For this review, take the finished solid that the model builds, in its own axes (mm). A direction names the side the tool comes from. Coordinates: 2 decimals unless noted, no trailing zeros. Write each loop counter-clockwise with the first axis right and the second up, starting at its lowest first coordinate (ties: lowest second). Pieces come first, ordered by that corner, then holes. Notation, with made-up numbers: M -2,16.5 L 30,16.5 A37 ccw 30,52.5 Z; hole C 23,79 d7. An arc over 180 degrees is marked long. One line per question, with ' | ' between items.
Autodesk Inventor part; units mm, degrees
ref_plane "Work Plane1" through (0, 0, -15) normal (0, 0, 1) x (1, 0, 0)
ref_plane "YZ Plane" through (0, 0, 0) normal (1, 0, 0) x (0, 1, 0)
ref_plane "XZ Plane" through (0, 0, 0) normal (0, 1, 0) x (-1, 0, 0)
sketch "Sketch1" plane through (0, 0, 0) normal (0, 0, 1) x (1, 0, 0)
  line L0 (0, 0) -> (25, 0)
  line L1 (25, 0) -> (25, 40)
  line L2 (25, 40) -> (0, 40)
  line L3 (0, 40) -> (0, 0)
  dimension "d1" = 25
  dimension "d2" = 40
  dimension "d3" = 25
extrude "Extrusion1" add sketch "Sketch1" against normal blind 30
sketch "Sketch2" plane through (25, 0, 0) normal (1, 0, 0) x (0, 0, -1)
  line L0 (0, 0) -> (30, 0)
  circle A0 centre (15, 6.56) radius 2.46
extrude "Extrusion2" cut sketch "Sketch2" against normal blind 30
sketch "Sketch3" plane through (0, 0, 0) normal (-1, 0, 0) x (0, 0, 1)
  line L0 (0, 0) -> (-30, 0)
  line L1 (-25.05, 0) -> (-4.95, 0)
  line L2 (-4.95, 0) -> (-4.95, 33.12)
  line L3 (-4.95, 33.12) -> (-25.05, 33.12)
  line L4 (-25.05, 33.12) -> (-25.05, 0)
  dimension "d11" = 20.1
extrude "Extrusion3" cut sketch "Sketch3" against normal blind 20
sketch "Sketch4" plane through (0, 0, 0) normal (0, -1, 0) x (1, 0, 0)
  line L0 (20, -4.95) -> (20, -25.05)
  line L1 (20, -15) -> (25, -15)
  line L2 (25, 0) -> (25, -30)
  line L3 (20, -8.025) -> (25, -8.025)
  line L4 (25, -8.025) -> (25, -21.975)
  line L5 (25, -21.975) -> (20, -21.975)
  line L6 (20, -21.975) -> (20, -8.025)
  line L7 (20, -8.025) -> (25, -21.975) construction
  line L8 (25, -8.025) -> (20, -21.975) construction
  line L9 (25, -12.54) -> (25, -17.46)
  point P0 (0, 0)
  point P1 (22.5, -15)
  dimension "d14" = 13.95
extrude "Extrusion4" add sketch "Sketch4" along normal blind 15
sketch "Sketch5" plane through (20, 0, 0) normal (-1, 0, 0) x (0, 0, 1)
  circle A0 centre (-15, 6.56) radius 2.46
  circle A1 centre (-15, 6.56) radius 4.7025
  circle A2 centre (-15, 6.56) radius 2.46
  circle A3 centre (-15, 6.56) radius 2.46
  point P0 (0, 0)
  dimension "d17" = 9.405
extrude "Extrusion5" cut sketch "Sketch5" against normal blind 2.1
sketch "Sketch6" plane through (25, 0, 0) normal (1, 0, 0) x (0, 0, -1)
  circle A0 centre (15, 6.56) radius 4.7025
  line L0 (15, 6.56) -> (15, 23.56)
  circle A1 centre (15, 23.56) radius 2.46
  point P0 (0, 0)
  dimension "d20" = 17
  dimension "d21" = 4.92
extrude "Extrusion6" cut sketch "Sketch6" against normal blind 10 contours A1
sketch "Sketch7" plane through (20, 0, 0) normal (-1, 0, 0) x (0, 0, 1)
  circle A0 centre (-15, 23.56) radius 2.46
  circle A1 centre (-15, 23.56) radius 4.7025
  point P0 (0, 0)
  dimension "d24" = 9.405
extrude "Extrusion7" cut sketch "Sketch7" against normal blind 2.1
sketch "Sketch9" plane through (25, 0, 0) normal (1, 0, 0) x (0, 0, -1)
  circle A0 centre (15, 6.56) radius 2.46
  circle A1 centre (15, 6.56) radius 2.46
  circle A2 centre (15, 23.56) radius 2.46
  circle A3 centre (15, 23.56) radius 2.46
  line L0 (30, 40) -> (30, 0)
  line L1 (30, 0) -> (30, 40)
  line L2 (30, 40) -> (0, 40)
  line L3 (0, 40) -> (0, 0)
  line L4 (0, 0) -> (8.025, 0)
  line L5 (21.975, 0) -> (21.975, -15)
  line L6 (21.975, -15) -> (8.025, -15)
  line L7 (8.025, -15) -> (8.025, 0)
  line L8 (0, 0) -> (8.025, 0)
  line L9 (21.975, 0) -> (30, 0)
extrude "Extrusion8" add sketch "Sketch9" along normal blind 5
sketch "Sketch10" plane through (0, 40, 0) normal (0, 1, 0) x (1, 0, 0)
  line L0 (0, 30) -> (30, 30)
  line L1 (30, 0) -> (0, 0)
  line L2 (0, 30) -> (30, 30)
  line L3 (30, 30) -> (30, 0)
  line L4 (30, 0) -> (0, 0)
  line L5 (0, 0) -> (0, 30)
extrude "Extrusion9" add sketch "Sketch10" along normal blind 30
sketch "Sketch12" plane through (30, 0, 0) normal (1, 0, 0) x (0, 0, -1)
  circle A0 centre (15, 6.56) radius 2.46
  line L0 (15, 6.56) -> (15, 15.06)
  circle A1 centre (15, 15.06) radius 2.525
  point P0 (0, 0)
  dimension "d31" = 8.5
  dimension "d33" = 5.05
extrude "Extrusion10" cut sketch "Sketch12" against normal blind 30 contours A1
sketch "Sketch14" plane through (0, 0, 0) normal (0, 0, 1) x (1, 0, 0)
  line L0 (30, 70) -> (0, 70)
  line L1 (0, 100) -> (-8, 100)
  line L2 (30, 0) -> (30, 70)
  line L3 (30, 118) -> (30, 70)
  line L4 (30, 105) -> (30, 100)
  line L5 (0, 70) -> (30, 70)
  line L6 (0, 70) -> (0, 100)
  line L7 (30, 122.5) -> (30, 118)
  line L8 (30, 70) -> (30, 145)
  line L9 (-2, 157.5) -> (-8, 160)
  line L10 (-2, 102.5) -> (-8, 100)
  line L11 (4, 130) -> (-2, 102.5)
  line L12 (4, 130) -> (-2, 157.5)
  line L13 (-8, 160) -> (15, 160)
  line L14 (30, 145) -> (15, 160)
  point P0 (0, 0)
  dimension "d47" = 30
extrude "Extrusion12" add sketch "Sketch14" against normal blind 30
sketch "Sketch15" plane through (0, 0, -25.05) normal (-1, 0, 0) x (0, 0, 1)
  line L0 (0, 33.12) -> (20.1, 33.12)
  line L1 (20.1, 33.12) -> (20.1, 0)
  line L2 (0, 33.12) -> (20.1, 33.12)
  line L3 (20.1, 33.12) -> (20.1, 31.1)
  line L4 (20.1, 31.1) -> (0, 31.1)
  line L5 (0, 31.1) -> (0, 33.12)
  point P0 (25.05, 0)
  dimension "d57" = 2.02
extrude "Extrusion13" add sketch "Sketch15" against normal blind 20
sketch "Sketch27" plane through (0, 0, 0) normal (0, 0, 1) x (1, 0, 0)
  point P0 (0, 0)
sketch "Sketch28" plane through (0, 0, 0) normal (0, 0, 1) x (1, 0, 0)
  line L0 (0, 100) -> (-8, 100)
  line L1 (0, 100) -> (-8, 100)
  line L2 (-8, 100) -> (-2, 102.5)
  line L3 (-8, 100) -> (-2, 102.5)
  line L4 (-2, 102.5) -> (4, 130)
  line L5 (-2, 102.5) -> (4, 130)
  line L6 (4, 130) -> (-2, 157.5)
  line L7 (4, 130) -> (-2, 157.5)
  line L8 (-2, 157.5) -> (-8, 160)
  line L9 (-2, 157.5) -> (-8, 160)
  line L10 (-8, 160) -> (15, 160)
  line L11 (-8, 160) -> (15, 160)
  line L12 (15, 160) -> (30, 145)
  line L13 (15, 160) -> (30, 145)
  line L14 (30, 145) -> (30, 93)
  line L15 (30, 0) -> (30, 145)
  line L16 (30, 93) -> (0, 93)
  line L17 (0, 0) -> (0, 100)
  line L18 (0, 93) -> (0, 100)
  dimension "d98" = 52
extrude "Extrusion14" add sketch "Sketch28" along normal blind 45
ref_plane "Work Plane1" through (0, 0, -15) normal (0, 0, 1) x (1, 0, 0)
mirror "Mirror1" about plane through (0, 0, -15) normal (0, 0, 1) of "Extrusion14"
properties part number "55mm_x_120mm"
1) We need section B-B on y = 6.56. State the section outline as (x, z) points.
Responses:
outline: M 0,-30 L 30,-30 L 30,-17.46 L 22.1,-17.46 L 22.1,-19.7 L 20,-19.7 L 20,-25.05 L 0,-25.05 Z; M 0,-4.95 L 20,-4.95 L 20,-10.3 L 22.1,-10.3 L 22.1,-12.54 L 30,-12.54 L 30,0 L 0,0 Z
2) To check wall thickness, follow line 1 along Z through (x, y) = (28.75, 23.56); line 2 along X through (y, z) = (75, -5.5); line 3 along Y through (x, z) = (14.5, -37). State the ranges of each line that lie inside material, in increasing order. Write a range as [from, to].
Responses:
line 1: [-30, -17.46], [-12.54, 0] | line 2: [0, 30] | line 3: [93, 160]
3) Machinability: for faces 4 (the flat face through (15, 47, -30)), 5 (the flat face through (15, 47, 0)), 6 (the flat face through (22.1, 21.5, -13)), 7 (the flat face through (-4.958, 101.268, -14.16)), 8 (the flat face through (20, 8, -20)), which of the approach directions +Z, -Z, +X, -X, +Y, -Y give a long, thin tool a straight path to every point of the face, cutting with its end or side? Answer none if there is none.
Responses:
face 4: -Z, +X, -X, -Y | face 5: +Z, +X, -X, -Y | face 6: -X | face 7: +Z, -Z, -X | face 8: -X, -Y
4) Insertion check: pin 1 Ø22 at (x, y) = (7.5, 17.5) entering from -Z; pin 2 Ø9 at (x, z) = (20.5, -2) entering from -Y; pin 3 Ø2 at (y, z) = (96, -61.5) entering from -X. Each pin has a flat end and moves straight along its axis. Give the tip position at first contact, or say it passes through.
Responses:
pin 1: z = -30 | pin 2: y = 0 | pin 3: x = 0
5) The part is to be moulded in two halves that separate along Y. For faces 1 (the flat face through (10, 31.1, -15)), 2 (the flat face through (-5.042, 158.768, -14.16)), 3 (the flat face through (10, 15, -4.95)), say which applies: +Y half, -Y half, draft (parallel to the pull), parting line (faces both ways), or undercut.
Responses:
face 1: -Y half | face 2: undercut | face 3: draft
6) We need section C-C on x = 26. State the section outline as (y, z) points (3 decimals).
Responses:
outline: M -15,-21.975 L 0,-21.975 L 0,-30 L 93,-30 L 93,-75 L 149,-75 L 149,45 L 93,45 L 93,0 L 0,0 L 0,-8.025 L -15,-8.025 Z; hole C 6.56,-15 d4.92; hole C 15.06,-15 d5.05; hole C 23.56,-15 d4.92
7) We need section D-D on x = 10.5. State the section outline as (y, z) points.
Responses:
outline: M 0,-30 L 93,-30 L 93,-75 L 160,-75 L 160,45 L 93,45 L 93,0 L 0,0 L 0,-4.95 L 31.1,-4.95 L 31.1,-25.05 L 0,-25.05 Z
8) We need section A-A on z = -15. State how many separate pieces and enclosed holes the cut face has, then the cut area to 3 significant figures.
Responses:
separate pieces: 4 | enclosed holes: 0 | area: 4,020 mm^2
